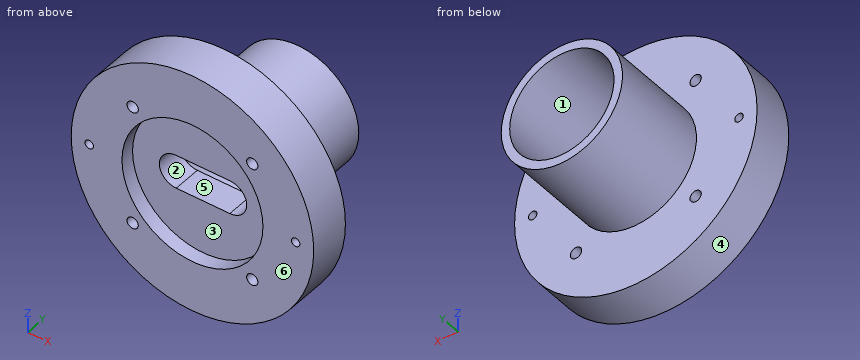
from build123d import *

# Parameters (mm, degrees)
SKETCH1_R             = 43
BOSS_EXTRUDE1_DEPTH   = 30
SKETCH6_R             = 25
CUT_EXTRUDE4_DEPTH    = 20
SKETCH10_R            = 21.5
SKETCH10_R_2          = 18.5
BOSS_EXTRUDE2_DEPTH   = 35
CUT_EXTRUDE6_DEPTH    = 31
F_3_0MM_DOWEL_HOLE1_D = 3
F_4_0MM_DOWEL_HOLE2_D = 4
SKETCH27_R            = 51.993622625
CUT_EXTRUDE7_DEPTH    = 15


with BuildPart() as part:
    # Sketch1 → Boss-Extrude1 (new body)
    with BuildSketch(Plane(origin=(0, 0, 0), x_dir=(1, 0, 0), z_dir=(0, 1, 0))):
        Circle(SKETCH1_R)
    extrude(amount=BOSS_EXTRUDE1_DEPTH)

    # Sketch6 → Cut-Extrude4 (cut)
    with BuildSketch(Plane.XZ):
        Circle(SKETCH6_R)
    extrude(amount=-CUT_EXTRUDE4_DEPTH, mode=Mode.SUBTRACT)

    # Sketch10 → Boss-Extrude2 (add)
    with BuildSketch(Plane(origin=(0, 30, 0), x_dir=(1, 0, 0), z_dir=(0, 1, 0))):
        Circle(SKETCH10_R)
        Circle(SKETCH10_R_2, mode=Mode.SUBTRACT)
    extrude(amount=BOSS_EXTRUDE2_DEPTH)

    # Sketch12 → Cut-Extrude6 (cut, through all)
    with BuildSketch(Plane(origin=(0, 30, 0), x_dir=(1, 0, 0), z_dir=(0, 1, 0))):
        with BuildLine():
            Line((-9.5, 6), (9.5, 6))
            ThreePointArc((9.5, 6), (15.5, 0), (9.5, -6))
            Line((9.5, -6), (-9.5, -6))
            ThreePointArc((-9.5, -6), (-15.5, 0), (-9.5, 6))
        make_face()
    extrude(amount=-CUT_EXTRUDE6_DEPTH, mode=Mode.SUBTRACT)

    # Ø3.0mm Dowel Hole1 (through all)
    with Locations(Plane(origin=(0, 30, 0), x_dir=(1, 0, 0), z_dir=(0, 1, 0))):
        with Locations((-36.6, 0), (36.6, 0)):
            Hole(F_3_0MM_DOWEL_HOLE1_D / 2)

    # Ø4.0mm Dowel Hole2 (through all)
    with Locations(Plane(origin=(0, 0, 0), x_dir=(-1, 0, 0), z_dir=(0, -1, 0))):
        with Locations((-21.213203436, -21.213203436), (21.213203436, -21.213203436), (-21.213203436, 21.213203436), (21.213203436, 21.213203436)):
            Hole(F_4_0MM_DOWEL_HOLE2_D / 2)

    # Sketch27 → Cut-Extrude7 (cut)
    with BuildSketch(Plane.XZ):
        Circle(SKETCH27_R)
    extrude(amount=-CUT_EXTRUDE7_DEPTH, mode=Mode.SUBTRACT)


solid = part.part
Could you check a few things on this model? Use its own coordinates, in mm. Face numbers are marked on the shaded views. A direction names the side the tool comes from. Coordinates: 2 decimals unless noted, no trailing zeros. Order: outer loops, then holes, each group sorted by start corner. A loop starts at its lowest first (then second) coordinate and runs counter-clockwise, first axis right, second up. Notation, with made-up numbers: (82, -3) - (100, -3) arc R23 cw to (100, 32) - close; hole circle Ø6 at (38.25, 22.25). An arc over 180 degrees is marked (long way). Answer in a Markdown table with one row per item. Add a question column.
(1) If we section it at C-C, the plane z = 16: Please give me the cut outline in (x, y).
(2) If we section it at B-B, the plane y = 49.5: Please give me the cut outline in (x, z).
(3) On a 3-axis mill with a long thin cutter (end or side, diameter ignored), from which of +Z, -Z, +X, -X, +Y, -Y can I reach the whole of each face in a straight line? I mean the marked faces 1, 2 and 3. Say none if no direction works.
(4) If we section it at D-D, the plane x = 11: Please give me the cut outline in (y, z), then the cut area to 3 significant figures.
(5) If we mould it in two halves opening along X, with no side actions, what happens to the marked faces 4, 5 and 6? For each: released by +X, released by -X, zero draft, split by the parting line, or undercut.
(6) Will these pins go through, and if not, where does the flat tip stop? pin 1 (11 mm diameter, centred on x = -1, y = 27, fed in from +Z); pin 2 (1.5 mm diameter, centred on x = -21.5, z = -11.5, fed in from +Y); pin 3 (1 mm diameter, centred on x = -32.5, y = 21.5, fed in from -Z); pin 4 (2.5 mm diameter, centred on x = 21.21, z = -21.21, fed in from +Y).
(7) If we section it at A-A, the plane x = 0: Please give me the cut outline in (y, z).
(8) I need wall thicknesses on L1, parallel to Y at x = -17, z = -4.5; L2, parallel to X at y = 52, z = 2; L3, parallel to Y at x = 24.5, z = -17. Which ranges of each line are inside material? Lowest first, please.
Results are:
| question | item | result |
|---|---|---|
| 1 | outline | (-39.91, 15) - (-19.21, 15) - (-19.21, 20) - (19.21, 20) - (19.21, 15) - (39.91, 15) - (39.91, 30) - (14.36, 30) - (14.36, 65) - (9.29, 65) - (9.29, 30) - (-9.29, 30) - (-9.29, 65) - (-14.36, 65) - (-14.36, 30) - (-39.91, 30) - close |
| 2 | outline | circle Ø43 at (0, 0); hole circle Ø37 at (0, 0) |
| 3 | face 1 | +Y |
| 3 | face 2 | +Y, -Y |
| 3 | face 3 | -Y |
| 4 | outline | (15, -41.57) - (30, -41.57) - (30, -18.47) - (65, -18.47) - (65, -14.87) - (30, -14.87) - (30, -5.81) - (20, -5.81) - (20, -22.45) - (15, -22.45) - close; (15, 22.45) - (20, 22.45) - (20, 5.81) - (30, 5.81) - (30, 14.87) - (65, 14.87) - (65, 18.47) - (30, 18.47) - (30, 41.57) - (15, 41.57) - close |
| 4 | area | 1,160 mm2 |
| 5 | face 4 | split by the parting line |
| 5 | face 5 | undercut |
| 5 | face 6 | zero draft |
| 6 | pin 1 | stops at z = 43 |
| 6 | pin 2 | stops at y = 30 |
| 6 | pin 3 | stops at z = -28.72 |
| 6 | pin 4 | passes through |
| 7 | outline | (15, -43) - (30, -43) - (30, -21.5) - (65, -21.5) - (65, -18.5) - (30, -18.5) - (30, -6) - (20, -6) - (20, -25) - (15, -25) - close; (15, 25) - (20, 25) - (20, 6) - (30, 6) - (30, 18.5) - (65, 18.5) - (65, 21.5) - (30, 21.5) - (30, 43) - (15, 43) - close |
| 8 | L1 | y = 20 to 30 |
| 8 | L2 | x = -21.41 to -18.39, 18.39 to 21.41 |
| 8 | L3 | y = 15 to 30 |
